```python
from build123d import *

# Parameters (mm, degrees)
F0_W      = 42.3
F0_H      = 42.3
F1_DEPTH  = 59
F2_R      = 11
F3_DEPTH  = 2
F4_R      = 2.5
F5_DEPTH  = 22
F7_DEPTH  = 15
F9_DEPTH  = 4.5
F10_DEPTH = 22
F11_DEPTH = 7


with BuildPart() as f1:
    # F0 (on Front) → F1 (new body)
    with BuildSketch(Plane.XZ):
        Rectangle(F0_W, F0_H)
    extrude(amount=F1_DEPTH)

    # F2 (on face) → F3 (join)
    with BuildSketch(Plane.XZ.offset(59)):
        Circle(F2_R)
    extrude(amount=F3_DEPTH)

    # F4 (on face) → F5 (join)
    with BuildSketch(Plane.XZ.offset(61)):
        Circle(F4_R)
    extrude(amount=F5_DEPTH)

    # F6 (on face) → F7 (cut)
    with BuildSketch(Plane.XZ.offset(83)):
        with BuildLine():
            ThreePointArc((0, 2.5), (-0.790569415, 2.3717082451), (-1.5, 2))
            Line((-1.5, 2), (0, 2))
            Line((0, 2), (0, 2.5))
        make_face()
        with BuildLine():
            Line((0, 2.5), (0, 2))
            Line((0, 2), (1.5, 2))
            ThreePointArc((1.5, 2), (0.790569415, 2.3717082451), (0, 2.5))
        make_face()
    extrude(amount=-F7_DEPTH, mode=Mode.SUBTRACT)

    # F8 (on face) → F9 (cut)
    with BuildSketch(Plane.XZ.offset(59)):
        with BuildLine():
            ThreePointArc((16.75, 15.5), (15.5, 16.75), (14.25, 15.5))
            Line((14.25, 15.5), (15.5, 15.5))
            Line((15.5, 15.5), (15.5, 14.25))
            ThreePointArc((15.5, 14.25), (16.3838834765, 14.6161165235), (16.75, 15.5))
        make_face()
        with BuildLine():
            Line((15.5, 15.5), (14.25, 15.5))
            ThreePointArc((14.25, 15.5), (14.6161165235, 14.6161165235), (15.5, 14.25))
            Line((15.5, 14.25), (15.5, 15.5))
        make_face()
        with BuildLine():
            Line((-15.5, 14.25), (-15.5, 15.5))
            Line((-15.5, 15.5), (-14.25, 15.5))
            ThreePointArc((-14.25, 15.5), (-16.3838834765, 16.3838834765), (-15.5, 14.25))
        make_face()
        with BuildLine():
            Line((-14.25, 15.5), (-15.5, 15.5))
            Line((-15.5, 15.5), (-15.5, 14.25))
            ThreePointArc((-15.5, 14.25), (-14.6161165235, 14.6161165235), (-14.25, 15.5))
        make_face()
        with BuildLine():
            Line((-15.5, -15.5), (-15.5, -14.25))
            ThreePointArc((-15.5, -14.25), (-16.3838834765, -16.3838834765), (-14.25, -15.5))
            Line((-14.25, -15.5), (-15.5, -15.5))
        make_face()
        with BuildLine():
            ThreePointArc((-14.25, -15.5), (-14.6161165235, -14.6161165235), (-15.5, -14.25))
            Line((-15.5, -14.25), (-15.5, -15.5))
            Line((-15.5, -15.5), (-14.25, -15.5))
        make_face()
        with BuildLine():
            Line((15.5, -15.5), (15.5, -14.25))
            ThreePointArc((15.5, -14.25), (14.6161165235, -14.6161165235), (14.25, -15.5))
            Line((14.25, -15.5), (15.5, -15.5))
        make_face()
        with BuildLine():
            ThreePointArc((16.75, -15.5), (16.3838834765, -14.6161165235), (15.5, -14.25))
            Line((15.5, -14.25), (15.5, -15.5))
            Line((15.5, -15.5), (14.25, -15.5))
            ThreePointArc((14.25, -15.5), (15.5, -16.75), (16.75, -15.5))
        make_face()
    extrude(amount=-F9_DEPTH, mode=Mode.SUBTRACT)

    # F10 (cut): a face of the model
    f10_faces = [f1.faces().sort_by_distance(p)[0] for p in [
        (0, -83, -0.120882785),
    ]]
    extrude(f10_faces, amount=-F10_DEPTH, mode=Mode.SUBTRACT)

    # F11 (cut): a face of the model
    f11_faces = [f1.faces().sort_by_distance(p)[0] for p in [
        (0, -68, 2.2018199305),
    ]]
    extrude(f11_faces, amount=-F11_DEPTH, mode=Mode.SUBTRACT)


solid = f1.part
```
Input: part model. Units: mm. Frame: model coordinates. A direction names the side the tool comes from. Give positions to 0.01 mm unless a question says otherwise; leave off trailing zeros. Order: outer loops, then holes, each group sorted by start corner. A loop starts at its lowest first (then second) coordinate and runs counter-clockwise, first axis right, second up.
1. Cut plane B-B (x = 0). Return loops of the section in (y, z), and give its area (3 significant figures).
Computed:
outline: (-61, -11) - (-59, -11) - (-59, -21.15) - (0, -21.15) - (0, 21.15) - (-59, 21.15) - (-59, 11) - (-61, 11) - close
area: 2,540 mm2
2. Line query: probe 1 along Z at (x, y) = (-15.5, -57.25); probe 2 along Z at (x, y) = (-15, -57). Output: solid intervals per line, ascending.
Computed:
probe 1: z = -21.15 to -16.75, -14.25 to 14.25, 16.75 to 21.15
probe 2: z = -21.15 to -16.65, -14.35 to 14.35, 16.65 to 21.15
3. Cut plane A-A (z = 0). Return loops of the section in (x, y).
Computed:
outline: (-21.15, -59) - (-11, -59) - (-11, -61) - (11, -61) - (11, -59) - (21.15, -59) - (21.15, 0) - (-21.15, 0) - close
4. Set-up query: faces 4 (the face through (0, 0, 0)), 5 (the face through (15, -54.5, -15)). Return all of +Z, -Z, +X, -X, +Y, -Y with unobstructed straight access to the full face (end or side cutting, diameter ignored); none if empty.
Computed:
face 4: +Z, -Z, +X, -X, +Y
face 5: -Y
5. Pin query (flat end, axial travel): pin 1 Ø2 at (x, z) = (-15.5, -15.5) entering from -Y; pin 2 Ø2 at (x, z) = (16, 16) entering from -Y. Return the tip coordinate at first contact, or that it passes through.
Computed:
pin 1: stops at y = -54.5
pin 2: stops at y = -59
6. Draft query along X for faces 1 (the face through (15, -54.5, 16)), 2 (the face through (-2.38, -59.99, -10.74)), 3 (the face through (-10, -59, -9)). Return one class per face: released by +X, released by -X, zero draft, split by the parting line, or undercut.
Computed:
face 1: undercut
face 2: split by the parting line
face 3: zero draft
